Autodesk Inventor part; units mm, degrees
ref_plane "YZ Plane" through (0, 0, 0) normal (1, 0, 0) x (0, 1, 0)
ref_plane "XZ Plane" through (0, 0, 0) normal (0, 1, 0) x (-1, 0, 0)
ref_plane "XY Plane" through (0, 0, 0) normal (0, 0, 1) x (1, 0, 0)
sketch "Sketch1" plane through (0, 0, 0) normal (0, 0, 1) x (1, 0, 0)
  line L0 (0, 0) -> (0, 50) construction
  line L1 (0, 0) -> (-30, 0)
  line L2 (-30, 0) -> (-30, 55)
  line L3 (-30, 55) -> (0, 55)
  line L4 (0, 55) -> (0, 50) construction
  line L5 (0, 50) -> (-25, 50)
  line L6 (-25, 50) -> (-25, 5)
  line L7 (-25, 5) -> (0, 5)
  line L8 (0, 5) -> (0, 0) construction
  line L9 (0, 0) -> (30, 0)
  line L10 (30, 0) -> (30, 55)
  line L11 (30, 55) -> (0, 55)
  line L12 (0, 50) -> (25, 50)
  line L13 (25, 50) -> (25, 5)
  line L14 (25, 5) -> (0, 5)
  dimension "d0" = 50
  dimension "d1" = 30
  dimension "d2" = 55
  dimension "d3" = 25
  dimension "d4" = 45
extrude "Extrusion1" add sketch "Sketch1" along normal blind 80
sketch "Sketch2" plane through (-30, 55, 0) normal (0, 1, 0) x (1, 0, 0)
  line L0 (13, -6) -> (47, -6)
  line L1 (47, -6) -> (47, -40)
  line L2 (47, -40) -> (13, -40)
  line L3 (13, -40) -> (13, -6)
  line L4 (13, -6) -> (47, -40) construction
  line L5 (47, -6) -> (13, -40) construction
  line L6 (14.5, -10) -> (45.5, -10)
  line L7 (45.5, -10) -> (45.5, -36)
  line L8 (45.5, -36) -> (14.5, -36)
  line L9 (14.5, -36) -> (14.5, -10)
  line L10 (14.5, -10) -> (45.5, -36) construction
  line L11 (45.5, -10) -> (14.5, -36) construction
  line L12 (0, 0) -> (0, -80)
  line L13 (60, 0) -> (0, 0)
  line L14 (60, -80) -> (0, -80)
  line L15 (60, 0) -> (60, -80)
  point P0 (30, 0)
  point P1 (30, -23)
  dimension "d7" = 34
  dimension "d8" = 34
  dimension "d9" = 31
  dimension "d10" = 26
  dimension "d11" = 30
  dimension "d12" = 23
extrude "Extrusion2" cut sketch "Sketch2" against normal blind 10 contours L6 L7 L8 L9
extrude "Extrusion3" add sketch "Sketch2" along normal blind 10 contours L0 L1 L2 L3
extrude "Extrusion4" add sketch "Sketch2" along normal blind 20 contours L13 L15 L14 L12
sketch "Sketch3" plane through (-30, 0, 0) normal (-1, 0, 0) x (0, 0, 1)
  line L0 (0, 0) -> (20, 0)
  line L1 (20, 0) -> (20, 35)
  line L2 (20, 35) -> (0, 35)
  line L3 (0, 35) -> (0, 0)
  dimension "d19" = 20
  dimension "d20" = 35
extrude "Extrusion5" cut sketch "Sketch3" against normal through all
sketch "Sketch4" plane through (-30, 65, 0) normal (0, 1, 0) x (1, 0, 0)
  line L0 (13, -40) -> (47, -40)
  line L1 (47, -40) -> (47, -6)
  line L2 (47, -6) -> (13, -6)
  line L3 (13, -6) -> (13, -40)
  line L4 (14.5, -36) -> (14.5, -10)
  line L5 (14.5, -10) -> (45.5, -10)
  line L6 (45.5, -10) -> (45.5, -36)
  line L7 (45.5, -36) -> (14.5, -36)
  point P0 (30, 0)
extrude "Extrusion6" add sketch "Sketch4" along normal blind 8
properties part number "color sensor holder"
Read the model definition and answer for the solid it produces. Units are mm, in the model's axes. A direction names the side the tool comes from. Round coordinates to 2 decimals unless told otherwise and drop trailing zeros. Write each loop counter-clockwise with the first axis right and the second up, starting at its lowest first coordinate (ties: lowest second). Pieces come first, ordered by that corner, then holes. Notation, with made-up numbers: (42.25, 78.5) - (99.25, 78.5) arc R9 ccw to (99.25, 90.5) - close; hole circle Ø11 at (63, 59.5). An arc over 180 degrees is marked (long way). One line per question, with ' | ' between items. Start each with the question number.
1. Find the intervals of material crossed by probe 1 along Y at (x, z) = (12.5, 67.5); probe 2 along X at (y, z) = (9.5, 62); probe 3 along Y at (x, z) = (-6.5, 39.5), in increasing order. Write a range as [from, to].
2. For a pull along Y with two mould halves and no side action, classify faces 6 (the face through (0, 50, 39)), 7 (the face through (27, 35, 10)), 8 (the face through (0, 59, 0)) as +Y half, -Y half, draft (parallel to the pull), parting line (faces both ways), or undercut.
3. For faces 1 (the face through (0, 61, 10)), 2 (the face through (2, 4, 20)), 3 (the face through (-25, 28, 48)), 4 (the face through (-30, 37, 39)), 5 (the face through (-17, 74, 23)), determine the directions among +Z, -Z, +X, -X, +Y, -Y from which every point of the face is accessible in a straight line to the end or side of a thin tool.
4. Section D-D (z = 55) is taken. Determine the outline of the cut face in (x, y).
5. Section B-B (z = 16) is taken. Determine the outline of the cut face in (x, y), and give its area (3 significant figures).
6. Section A-A (y = 16.5) is taken. Determine the outline of the cut face in (x, z), and give its area (3 significant figures).
7. This flat-tipped pin is pushed along its axis until it touches: pin 1 (2.5 mm diameter, centred on x = 26.5, z = 7.5, fed in from -Y). Where does it stop, or does it pass through?
8. Section C-C (x = 18.5) is taken. Determine the outline of the cut face in (y, z), and give its area (3 significant figures).
Filled in:
1) probe 1: [0, 5], [50, 75] | probe 2: [-30, -25], [25, 30] | probe 3: [0, 5], [50, 73]
2) face 6: undercut | face 7: -Y half | face 8: draft
3) face 1: +Y, -Y | face 2: -Z, +X, -X, -Y | face 3: +Z, -Z | face 4: +Z, -Z, -X, +Y, -Y | face 5: +Y
4) outline: (-30, 0) - (30, 0) - (30, 75) - (-30, 75) - close; hole (-25, 5) - (25, 5) - (25, 50) - (-25, 50) - close
5) outline: (-30, 35) - (-25, 35) - (-25, 50) - (-15.5, 50) - (-15.5, 73) - (-17, 73) - (-17, 75) - (-30, 75) - close; (15.5, 50) - (25, 50) - (25, 35) - (30, 35) - (30, 75) - (17, 75) - (17, 73) - (15.5, 73) - close | area: 869 mm²
6) outline: (-30, 20) - (-25, 20) - (-25, 80) - (-30, 80) - close; (25, 20) - (30, 20) - (30, 80) - (25, 80) - close | area: 600 mm²
7) pin 1: y = 35
8) outline: (0, 20) - (5, 20) - (5, 80) - (0, 80) - close; (50, 0) - (75, 0) - (75, 80) - (50, 80) - close | area: 2,300 mm²
